Build history of the part. All positions in model axes, mm. A direction names the side the tool comes from. Round coordinates to 2 decimals unless told otherwise and drop trailing zeros. Write each loop counter-clockwise with the first axis right and the second up, starting at its lowest first coordinate (ties: lowest second). Pieces come first, ordered by that corner, then holes. Notation, with made-up numbers: M -15.75,57.25 L 4.25,57.25 A20 ccw 4.25,69.25 Z; hole C 71.5,10.25 d5. An arc over 180 degrees is marked long. Write item = value, one per line.
from build123d import *

# Parameters (mm, degrees)
BOSS_EXTRUDE1_DEPTH = 22
SKETCH2_R           = 3.75
CUT_EXTRUDE1_DEPTH  = 5
SKETCH3_R           = 2.4
CUT_EXTRUDE2_DEPTH  = 5
SKETCH4_R           = 3.75
CUT_EXTRUDE3_DEPTH  = 5
SKETCH5_R           = 2.4
CUT_EXTRUDE4_DEPTH  = 5
CHAMFER1_SIZE       = 20


with BuildPart() as part:
    # Sketch1 → Boss-Extrude1 (new body)
    with BuildSketch(Plane(origin=(0, 0, 0), x_dir=(0, 0, -1), z_dir=(1, 0, 0))):
        Polygon((0, 0), (-42, 0), (-42, -8), (8, -8), (8, 42), (0, 42), align=None)
    extrude(amount=BOSS_EXTRUDE1_DEPTH)

    # Sketch2 → Cut-Extrude1 (cut)
    with BuildSketch(Plane.XY):
        with Locations((11, 34)):
            Circle(SKETCH2_R)
    extrude(amount=-CUT_EXTRUDE1_DEPTH, mode=Mode.SUBTRACT)

    # Sketch3 → Cut-Extrude2 (cut)
    with BuildSketch(Plane.XY.offset(-5)):
        with Locations((11, 34)):
            Circle(SKETCH3_R)
    extrude(amount=-CUT_EXTRUDE2_DEPTH, mode=Mode.SUBTRACT)

    # Sketch4 → Cut-Extrude3 (cut)
    with BuildSketch(Plane(origin=(0, 0, 0), x_dir=(1, 0, 0), z_dir=(0, 1, 0))):
        with Locations(Location((11, -34, 0), (0, 0, 270))):
            Circle(SKETCH4_R)
    extrude(amount=-CUT_EXTRUDE3_DEPTH, mode=Mode.SUBTRACT)

    # Sketch5 → Cut-Extrude4 (cut)
    with BuildSketch(Plane(origin=(0, -5, 0), x_dir=(1, 0, 0), z_dir=(0, 1, 0))):
        with Locations(Location((11, -34, 0), (0, 0, 270))):
            Circle(SKETCH5_R)
    extrude(amount=-CUT_EXTRUDE4_DEPTH, mode=Mode.SUBTRACT)

    # Chamfer1
    chamfer1_edges = [part.edges().sort_by_distance(p)[0] for p in [
        (11, 0, 0),
    ]]
    chamfer(chamfer1_edges, length=CHAMFER1_SIZE)


solid = part.part
1. Probe probe 1 along X at (y, z) = (-1.3, 34); probe 2 along Y at (x, z) = (11, -6); probe 3 along X at (y, z) = (-6.05, 34). List the from-to ranges inside material, lowest first.
Responses:
probe_1 = 0 to 7.25, 14.75 to 22
probe_2 = -8 to 31.6, 36.4 to 42
probe_3 = 0 to 8.6, 13.4 to 22
2. Band-saw the part on D-D (x = 20). List the corners of the cut face in (y, z), plus the area to 3 significant figures.
Responses:
outline = M -8,-8 L 42,-8 L 42,0 L 20,0 L 0,20 L 0,42 L -8,42 Z
area = 936 mm²
3. Band-saw the part on C-C (x = 11). List the corners of the cut face in (y, z).
Responses:
outline = M -8,-8 L 31.6,-8 L 31.6,-5 L 30.25,-5 L 30.25,0 L 20,0 L 0,20 L 0,30.25 L -5,30.25 L -5,31.6 L -8,31.6 Z; M -8,36.4 L -5,36.4 L -5,37.75 L 0,37.75 L 0,42 L -8,42 Z; M 36.4,-8 L 42,-8 L 42,0 L 37.75,0 L 37.75,-5 L 36.4,-5 Z
4. Band-saw the part on A-A (y = 34). List the corners of the cut face in (x, z).
Responses:
outline = M 0,-8 L 8.6,-8 L 8.6,-5 L 7.25,-5 L 7.25,0 L 0,0 Z; M 13.4,-8 L 22,-8 L 22,0 L 14.75,0 L 14.75,-5 L 13.4,-5 Z
5. Mould opens along Y. For faces 4 (the face through (11, 17, -8)), 5 (the face through (11, -8, 17)), 6 (the face through (13.45, 33.22, -5)) say: pulls with the +Y half, pulls with the -Y half, needs draft (parallel to the pull), parting line crosses it, or undercut.
Responses:
face_4 = needs draft
face_5 = pulls with the -Y half
face_6 = undercut
6. Tool access for faces 1 (the face through (8.024, 31.718, -2.465)), 2 (the face through (8.55, -5, 34.78)), 3 (the face through (11, 0, 28)): list every direction of +Z, -Z, +X, -X, +Y, -Y with a clear straight run to the whole face (end or side of a thin tool).
Responses:
face_1 = +Z
face_2 = +Y
face_3 = +Z, +X, -X, +Y
7. Flat gauge pins, fed straight in: pin 1 (10 mm diameter, centred on x = 10.5, z = 26.5, fed in from +Y); pin 2 (6 mm diameter, centred on x = 11, y = 34, fed in from +Z); pin 3 (4 mm diameter, centred on x = 11, y = 36, fed in from +Z). Where does each tip first touch, or does it go through?
Responses:
pin_1 = 0
pin_2 = -5
pin_3 = 0
